```python
from build123d import *

# Parameters (mm, degrees)
SKETCH_2_W             = 11
SKETCH_2_H             = 11
CUT_EXTRUDE_1_DEPTH    = 1
FILLET_1_R             = 2
SKETCH_5_R             = 7.5
SKETCH_5_R_2           = 5.25
EXTRUDE_1_DEPTH        = 3.5
SKETCH_6_R             = 1.25
CUT_EXTRUDE_M3_1_DEPTH = 40.799497484
CHAMFER_1_SIZE         = 0.5
CUT_EXTRUDE_M3_REACH   = 44.335
SKETCH_7_R             = 1.25
CHAMFER_2_SIZE         = 1
CUT_EXTRUDE_14_DEPTH   = 3.5
FILLET_2_R             = 2.25


with BuildPart() as part:
    # 草图1 → 旋转1 (revolve)
    with BuildSketch(Plane(origin=(0, 0, 0), x_dir=(0, 0, -1), z_dir=(1, 0, 0))):
        Polygon((-7.5, 0), (-5.25, 0), (-5.25, 18), (0, 18), (0, 28), (-20, 28), (-20, 21), (-9, 21), (-9, 18), (-7.5, 18), align=None)
    revolve(axis=Axis((0, 28, 0), (0, -1, 0)))

    # 草图2 → 切除-拉伸1 (cut)
    with BuildSketch(Plane(origin=(0, 28, 0), x_dir=(1, 0, 0), z_dir=(0, 1, 0))):
        Rectangle(SKETCH_2_W, SKETCH_2_H)
    extrude(amount=-CUT_EXTRUDE_1_DEPTH, mode=Mode.SUBTRACT)

    # 圆角1
    fillet_1_edges = [part.edges().sort_by_distance(p)[0] for p in [
        (5.5, 27.5, -5.5),
        (5.5, 27.5, 5.5),
        (-5.5, 27.5, 5.5),
        (-5.5, 27.5, -5.5),
    ]]
    fillet(fillet_1_edges, radius=FILLET_1_R)

    # 草图5 → 凸台-拉伸1 (add)
    with BuildSketch(Plane.XZ):
        with Locations(Location((0, 0, 0), (0, 0, 90))):
            Circle(SKETCH_5_R)
        with Locations(Location((0, 0, 0), (0, 0, 90))):
            Circle(SKETCH_5_R_2, mode=Mode.SUBTRACT)
    extrude(amount=EXTRUDE_1_DEPTH)

    # 草图6 → M3螺纹孔1 (cut, through all)
    with BuildSketch(Plane.XY):
        with Locations((0, 7.5)):
            Circle(SKETCH_6_R)
    extrude(amount=-CUT_EXTRUDE_M3_1_DEPTH, mode=Mode.SUBTRACT)

    # 倒角1
    chamfer_1_edges = [part.edges().sort_by_distance(p)[0] for p in [
        (0, -3.5, -7.5),
        (0, 18, -9),
    ]]
    chamfer(chamfer_1_edges, length=CHAMFER_1_SIZE)

    # 草图7 → M3螺纹孔 (cut, up to next)
    with BuildSketch(Plane(origin=(0, 28, 0), x_dir=(1, 0, 0), z_dir=(0, 1, 0)), mode=Mode.PRIVATE) as cut_extrude_m3_sk1:
        with Locations(Location((0, 16, 0), (0, 0, 270))):
            Circle(SKETCH_7_R)
    cut_extrude_m3_tool1 = extrude(cut_extrude_m3_sk1.sketch, amount=-CUT_EXTRUDE_M3_REACH, mode=Mode.PRIVATE) & part.part
    # 草图7 → M3螺纹孔 (cut, up to next)
    with BuildSketch(Plane(origin=(0, 28, 0), x_dir=(1, 0, 0), z_dir=(0, 1, 0)), mode=Mode.PRIVATE) as cut_extrude_m3_sk2:
        with Locations(Location((16, 0, 0), (0, 0, 270))):
            Circle(SKETCH_7_R)
    cut_extrude_m3_tool2 = extrude(cut_extrude_m3_sk2.sketch, amount=-CUT_EXTRUDE_M3_REACH, mode=Mode.PRIVATE) & part.part
    # 草图7 → M3螺纹孔 (cut, up to next)
    with BuildSketch(Plane(origin=(0, 28, 0), x_dir=(1, 0, 0), z_dir=(0, 1, 0)), mode=Mode.PRIVATE) as cut_extrude_m3_sk3:
        with Locations(Location((0, -16, 0), (0, 0, 270))):
            Circle(SKETCH_7_R)
    cut_extrude_m3_tool3 = extrude(cut_extrude_m3_sk3.sketch, amount=-CUT_EXTRUDE_M3_REACH, mode=Mode.PRIVATE) & part.part
    # 草图7 → M3螺纹孔 (cut, up to next)
    with BuildSketch(Plane(origin=(0, 28, 0), x_dir=(1, 0, 0), z_dir=(0, 1, 0)), mode=Mode.PRIVATE) as cut_extrude_m3_sk4:
        with Locations(Location((-16, 0, 0), (0, 0, 270))):
            Circle(SKETCH_7_R)
    cut_extrude_m3_tool4 = extrude(cut_extrude_m3_sk4.sketch, amount=-CUT_EXTRUDE_M3_REACH, mode=Mode.PRIVATE) & part.part
    add(cut_extrude_m3_tool1.solids().sort_by_distance((0, 28, -16))[0], mode=Mode.SUBTRACT)
    add(cut_extrude_m3_tool2.solids().sort_by_distance((16, 28, 0))[0], mode=Mode.SUBTRACT)
    add(cut_extrude_m3_tool3.solids().sort_by_distance((0, 28, 16))[0], mode=Mode.SUBTRACT)
    add(cut_extrude_m3_tool4.solids().sort_by_distance((-16, 28, 0))[0], mode=Mode.SUBTRACT)

    # 倒角2
    chamfer_2_edges = [part.edges().sort_by_distance(p)[0] for p in [
        (0, 28, -20),
        (0, 21, -20),
    ]]
    chamfer(chamfer_2_edges, length=CHAMFER_2_SIZE)

    # 草图8 → 切除-拉伸14 (cut)
    with BuildSketch(Plane.XZ.offset(-21)):
        with BuildLine():
            Line((-9.866772518, 3.591211505), (-14.095389312, 5.13030215))
            ThreePointArc((-14.095389312, 5.13030215), (0, -15), (14.095389312, 5.13030215))
            Line((14.095389312, 5.13030215), (9.866772518, 3.591211505))
            ThreePointArc((9.866772518, 3.591211505), (0, -10.5), (-9.866772518, 3.591211505))
        make_face()
    extrude(amount=-CUT_EXTRUDE_14_DEPTH, mode=Mode.SUBTRACT)

    # 圆角2
    fillet_2_edges = [part.edges().sort_by_distance(p)[0] for p in [
        (9.866772518, 22.75, 3.591211505),
        (14.095389312, 22.75, 5.13030215),
        (-9.866772518, 22.75, 3.591211505),
        (-14.095389312, 22.75, 5.13030215),
    ]]
    fillet(fillet_2_edges, radius=FILLET_2_R - 0.0001)  # a hair under: the kernel refuses the full size


solid = part.part
```
Check sheet for the modelled part. Datum: model origin and axes. Units: mm. A direction names the side the tool comes from. Coordinates: 2 decimals unless noted, no trailing zeros. Write each loop counter-clockwise with the first axis right and the second up, starting at its lowest first coordinate (ties: lowest second). Pieces come first, ordered by that corner, then holes. Notation, with made-up numbers: M 23.25,-9 L 41.25,-9 A22 cw 41.25,5 Z; hole C 3,20.5 d11. An arc over 180 degrees is marked long. Write item = value, one per line. Start each with the question number.
1. Sectioned sample at B-B (y = 2.5). Record the cut outline in (x, z).
2. Mould release check, pull along Z, two halves, no side actions. Record for faces 1 (the cylindrical face through (-13.666, 22.774, 4.139)), 2 (the cylindrical face through (2.87, 7.35, 6.93)), 3 (the flat face through (-5, -3.5, 3)): pulls with the +Z half, pulls with the -Z half, needs draft (parallel to the pull), parting line crosses it, or undercut.
3. Go/stop test with flat-tipped pins: pin 1 (1 mm diameter, centred on y = 16, z = 9.5, fed in from -X); pin 2 (4 mm diameter, centred on x = 0, z = -16, fed in from -Y); pin 3 (0.5 mm diameter, centred on y = 27.5, z = -1, fed in from -X) (3 decimals); pin 4 (9 mm diameter, centred on x = -0.5, z = 0, fed in from +Y). Record where each tip stops, or that it passes through.
4. Sectioned sample at C-C (y = 7.5). Record the cut outline in (x, z).
5. Sectioned sample at A-A (z = 0). State how many separate pieces and enclosed holes the cut face has, then the cut area to 4 significant figures.
6. Thickness scan on probe 1 along X at (y, z) = (23, 0); probe 2 along X at (y, z) = (9.75, 0); probe 3 along X at (y, z) = (25, -16). Record the ranges inside material, lowest first.
7. Tool access check on faces 4 (the cylindrical face through (-17.22, 24.55, -0.27)), 5 (the cylindrical face through (4.93, 27.49, -4.9)), 6 (the cylindrical face through (10.627, 22.774, 3.325)). Record the directions out of +Z, -Z, +X, -X, +Y, -Y that give a thin tool (end or side, any length) a straight path to the whole face; none if there is none.
The answers:
q1.outline = C 0,0 d15; hole C 0,0 d10.5
q2.face_1 = undercut
q2.face_2 = parting line crosses it
q2.face_3 = needs draft
q3.pin_1 = through
q3.pin_2 = 21
q3.pin_3 = -19.725
q3.pin_4 = 27
q4.outline = M -1.25,-7.4 L -1.25,-5.1 A5.25 cw long 1.25,-5.1 L 1.25,-7.4 A7.5 ccw long Z
q5.separate_pieces = 3
q5.enclosed_holes = 0
q5.area = 352.5 mm²
q6.probe_1 = -20 to -17.25, -10.5 to 10.5, 17.25 to 20
q6.probe_2 = -7.5 to -5.25, 5.25 to 7.5
q6.probe_3 = -12 to -1.25, 1.25 to 12
q7.face_4 = +Y, -Y
q7.face_5 = +Y
q7.face_6 = -Y
